The listing builds one solid part. Answer for the finished solid, in the listing's coordinates (mm). A direction names the side the tool comes from. Coordinates: 2 decimals unless noted, no trailing zeros. Order: outer loops, then holes, each group sorted by start corner. A loop starts at its lowest first (then second) coordinate and runs counter-clockwise, first axis right, second up. Notation, with made-up numbers: (48, 45.25) -> (105, 45.25) arc R19 ccw to (105, 76.25) -> close; hole circle Ø6 at (14.5, 33). An arc over 180 degrees is marked (long way). Return JSON: item names as keys, results as strings.
from build123d import *

# Parameters (mm, degrees)
F1_DEPTH = 6
F2_R     = 3
F3_DEPTH = 0.5
F4_R     = 3
F5_DEPTH = 0.5
F6_R     = 2.99999
F7_R     = 2.99999
F9_DEPTH = 1
F10_R    = 3
F11_R    = 2.99999


# Not quite as in the source:
# - a fillet or chamfer is up to 0.001 mm smaller than in the source, because OpenCascade refuses the exact size


with BuildPart() as f1:
    # F0 (on Top) → F1 (new body)
    with BuildSketch(Plane.XY):
        with BuildLine():
            Line((-3.15, 8.1), (-3.15, 10.1734949747))
            ThreePointArc((-3.15, 10.1734949747), (-5.6194604457, 9.046776459), (-7.7238904562, 7.3323949854))
            ThreePointArc((-7.7238904562, 7.3323949854), (0, -10.65), (7.7238904562, 7.3323949854))
            ThreePointArc((7.7238904562, 7.3323949854), (5.6194604457, 9.046776459), (3.15, 10.1734949747))
            Line((3.15, 10.1734949747), (3.15, 8.1))
            Line((3.15, 8.1), (0, 8.1))
            Line((0, 8.1), (-3.15, 8.1))
        make_face()
        with BuildLine():
            ThreePointArc((3.15, 0), (-2.2273863607, -2.2273863607), (0, 3.15))
            ThreePointArc((0, 3.15), (2.2273863607, 2.2273863607), (3.15, 0))
        make_face(mode=Mode.SUBTRACT)
        with BuildLine():
            ThreePointArc((-7.7238904562, 7.3323949854), (-5.6194604457, 9.046776459), (-3.15, 10.1734949747))
            Line((-3.15, 10.1734949747), (-3.15, 23.35))
            Line((-3.15, 23.35), (-9.6377339195, 19.5871143267))
            Line((-9.6377339195, 19.5871143267), (-9.6377339195, 10.6575252249))
            ThreePointArc((-9.6377339195, 10.6575252249), (-8.1670066914, 9.2906908645), (-7.7238904562, 7.3323949854))
        make_face()
        with BuildLine():
            ThreePointArc((3.15, 10.1734949747), (5.6194604457, 9.046776459), (7.7238904562, 7.3323949854))
            ThreePointArc((7.7238904562, 7.3323949854), (8.1670066914, 9.2906908645), (9.6377339195, 10.6575252249))
            Line((9.6377339195, 10.6575252249), (9.6377339195, 19.5871143267))
            Line((9.6377339195, 19.5871143267), (3.15, 23.35))
            Line((3.15, 23.35), (3.15, 10.1734949747))
        make_face()
    extrude(amount=F1_DEPTH)

    # F2 (on face) → F3 (join)
    with BuildSketch(Plane.YZ.offset(-3.15)):
        with Locations((18.85, 3)):
            Circle(F2_R)
    extrude(amount=F3_DEPTH)

    # F4 (on face) → F5 (join)
    with BuildSketch(Plane(origin=(3.15, 0, 0), x_dir=(0, -1, 0), z_dir=(-1, 0, 0))):
        with Locations((-18.85, 3)):
            Circle(F4_R)
    extrude(amount=F5_DEPTH)

    # F6 (radius 3 in the source; OpenCascade refuses exactly that, so slightly less here)
    f6_edges = [f1.edges().sort_by_distance(p)[0] for p in [
        (-6.393867, 21.468557, 0),
        (-6.393867, 21.468557, 6),
    ]]
    fillet(f6_edges, radius=F6_R)

    # F7 (radius 3 in the source; OpenCascade refuses exactly that, so slightly less here)
    f7_edges = [f1.edges().sort_by_distance(p)[0] for p in [
        (6.393867, 21.468557, 0),
        (6.393867, 21.468557, 6),
    ]]
    fillet(f7_edges, radius=F7_R)

    # F8 (on face) → F9 (cut)
    with BuildSketch(Plane.XY.offset(6)):
        Polygon((-0.5410675658, -4.1934514275), (-0.2322952287, -4.1934514275), (-1.4496098506, -6.0194233604), (-2.6669244725, -4.1934514275), (-2.3, -4.1934514275), (-2.3, -3.9827399887), (-3.5, -3.9827399887), (-3.5, -4.1934514275), (-3.1341812573, -4.1934514275), (-2.8992197012, -4.5418942706), (-1.6819050793, -6.3678662034), (-3.0600394749, -8.4350677969), (-3.1399389263, -8.5422809794), (-3.5, -8.5422809794), (-3.5, -8.7529924182), (-2.3, -8.7529924182), (-2.3, -8.5422809794), (-2.6669244725, -8.5422809794), (-1.4496098506, -6.7163090465), (-0.2322952287, -8.5422809794), (-0.5410675658, -8.5422809794), (-0.5410675658, -8.7529924182), (0.5013382179, -8.7529924182), (0.5013382179, -8.5422809794), (0.2322952287, -8.5422809794), (1.4496098506, -6.7163090465), (2.6669244725, -8.5422809794), (2.3810260464, -8.5422809794), (2.3810260464, -8.7529924182), (3.4986780956, -8.7529924182), (3.5, -8.5422809794), (3.1424169429, -8.5422809794), (3.0600394749, -8.4350677969), (1.6819050793, -6.3678662034), (2.8992197012, -4.5418942706), (3.1315149299, -4.1934514275), (3.3579636365, -4.1934514275), (3.5, -4.1934514275), (3.4986780956, -3.9827399887), (2.3810260464, -3.9827399887), (2.3810260464, -4.1934514275), (2.6669244725, -4.1934514275), (1.4496098506, -6.0194233604), (0.1581401168, -4.1934514275), (0.5013382179, -4.1934514275), (0.5013382179, -3.9827399887), (-0.5410675658, -3.9827399887), align=None)
        Polygon((-1.2173146219, -6.3678662034), (0, -4.5418942706), (1.2173146219, -6.3678662034), (0, -8.1938381363), align=None, mode=Mode.SUBTRACT)
    extrude(amount=-F9_DEPTH, mode=Mode.SUBTRACT)

    # F10
    f10_edges = [f1.edges().sort_by_distance(p)[0] for p in [
        (0, 8.1, 6),
    ]]
    fillet(f10_edges, radius=F10_R)

    # F11 (radius 3 in the source; OpenCascade refuses exactly that, so slightly less here)
    f11_edges = [f1.edges().sort_by_distance(p)[0] for p in [
        (0, 8.1, 0),
    ]]
    fillet(f11_edges, radius=F11_R)


solid = f1.part
1. The part is cut by section A-A on y = 14. Give the vertices of the cut face in (x, z), and give its area (3 significant figures).
Answer block:
{"outline": "(-9.64, 0) -> (-3.15, 0) -> (-3.15, 6) -> (-9.64, 6) -> close; (3.15, 0) -> (9.64, 0) -> (9.64, 6) -> (3.15, 6) -> close", "area": "77.9 mm2"}
2. Consider line 1 (X direction, y = 11, z = 1.05); line 2 (Y direction, x = -9.25, z = 4.3); line 3 (Y direction, x = 0, z = 4.7). Determine where each line is inside the solid, lowest interval first. Write a range as from..to.
Answer block:
{"line 1": "x = -9.64..-3.15, 3.15..9.64", "line 2": "y = -5.28..5.28, 10.44..19.47", "line 3": "y = -10.65..-3.15, 3.15..7.57"}
3. Each of these flat-tipped pins is pushed along its axis until it touches: pin 1 Ø3 at (x, z) = (-4.5, 1.5) entering from -Y; pin 2 Ø3.5 at (y, z) = (20.5, 4) entering from +X; pin 3 Ø10 at (x, y) = (0.5, 14.5) entering from -Z; pin 4 Ø1.1 at (x, z) = (3, 5.5) entering from +Y. Where does it stop, or does it pass through?
Answer block:
{"pin 1": "stops at y = -10.22", "pin 2": "stops at x = 9.64", "pin 3": "stops at z = 0", "pin 4": "stops at y = 22.5"}
4. Determine the mould class of faces 6 (the face through (-6.75, 20.219, 0.855)), 7 (the face through (2.9, -3.983, 5.5)), 8 (the face through (-2.3, -5.44, 5.51)), 9 (the face through (9.638, 15, 3)) for opening direction Y: pulls with the +Y half, pulls with the -Y half, needs draft (parallel to the pull), parting line crosses it, or undercut.
Answer block:
{"face 6": "pulls with the +Y half", "face 7": "undercut", "face 8": "undercut", "face 9": "needs draft"}
5. The part is cut by section C-C on z = 3.8. Give the vertices of the cut face in (x, y), and give its area (3 significant figures).
Answer block:
{"outline": "(-9.64, 10.66) arc R3.4 cw to (-7.72, 7.33) arc R10.65 ccw (long way) to (7.72, 7.33) arc R3.4 cw to (9.64, 10.66) -> (9.64, 19.46) -> (3.15, 23.22) -> (3.15, 21.74) -> (2.65, 21.74) -> (2.65, 15.96) -> (3.15, 15.96) -> (3.15, 7.99) -> (-3.15, 7.99) -> (-3.15, 15.96) -> (-2.65, 15.96) -> (-2.65, 21.74) -> (-3.15, 21.74) -> (-3.15, 23.22) -> (-9.64, 19.46) -> close; hole circle Ø6.3 at (0, 0)", "area": "472 mm2"}
6. For faces 1 (the face through (-2.65, 19, 3)), 2 (the face through (-0.04, 7.2, 0.86)), 3 (the face through (-8.181, 9.315, 2.958)), 4 (the face through (2.9, 21.06, 5.03)), 5 (the face through (-2.9, -3.983, 5.5)), determine the directions among +Z, -Z, +X, -X, +Y, -Y from which every point of the face is accessible in a straight line to the end or side of a thin tool.
Answer block:
{"face 1": "+Z, -Z, +Y", "face 2": "-Z", "face 3": "+Z, -Z, -X", "face 4": "none", "face 5": "+Z"}
7. The part is cut by section D-D on y = -3.5. Give the vertices of the cut face in (x, z), and give its area (3 significant figures).
Answer block:
{"outline": "(-10.06, 0) -> (10.06, 0) -> (10.06, 6) -> (-10.06, 6) -> close", "area": "121 mm2"}
8. The part is cut by section B-B on z = 2.1. Give the vertices of the cut face in (x, y), and give its area (3 significant figures).
Answer block:
{"outline": "(-9.64, 10.66) arc R3.4 cw to (-7.72, 7.33) arc R10.65 ccw (long way) to (7.72, 7.33) arc R3.4 cw to (9.64, 10.66) -> (9.64, 19.43) -> (3.15, 23.19) -> (3.15, 21.71) -> (2.65, 21.71) -> (2.65, 15.99) -> (3.15, 15.99) -> (3.15, 7.96) -> (-3.15, 7.96) -> (-3.15, 15.99) -> (-2.65, 15.99) -> (-2.65, 21.71) -> (-3.15, 21.71) -> (-3.15, 23.19) -> (-9.64, 19.43) -> close; hole circle Ø6.3 at (0, 0)", "area": "471 mm2"}
